from build123d import *

# Parameters (mm, degrees)
BOSS_EXTRUDE1_DEPTH = 4
SKETCH6_R           = 1.45
CUT_EXTRUDE1_DEPTH  = 63.610622102
SKETCH7_R           = 1.4
CUT_EXTRUDE2_DEPTH  = 64.549114864
FILLET1_R           = 1
FILLET2_R           = 0.5


with BuildPart() as part:
    # Sketch4 → Revolve1 (revolve)
    with BuildSketch(Plane(origin=(0, 0, 0), x_dir=(1, 0, 0), z_dir=(0, 1, 0)), mode=Mode.PRIVATE) as revolve1_sk:
        Polygon((9.95, -8.8), (0, -8.8), (0, 0), (12.5, 0), (12.5, -0.8), (11.5, -1.8), (9.95, -1.8), align=None)
    revolve1 = revolve(revolve1_sk.sketch.rotate(Axis((0, 0, 0), (0, 0, 1)), 180), axis=Axis((0, 0, 0), (0, 0, 1)))

    # Sketch5 → Boss-Extrude1 (add)
    with BuildSketch(Plane.XY):
        with BuildLine():
            Line((0, 12.5), (-60, 12.5))
            Line((-60, 12.5), (-60, -12.5))
            Line((-60, -12.5), (0, -12.5))
            ThreePointArc((0, -12.5), (12.5, 0), (0, 12.5))
        make_face()
    boss_extrude1 = extrude(amount=-BOSS_EXTRUDE1_DEPTH)

    # Sketch6 → Cut-Extrude1 (cut, through all)
    with BuildSketch(Plane.XY.offset(8.8)):
        with Locations((0, 6.5)):
            Circle(SKETCH6_R)
        with Locations((6.5, 0)):
            Circle(SKETCH6_R)
        with Locations((0, -6.5)):
            Circle(SKETCH6_R)
        with Locations((-6.5, 0)):
            Circle(SKETCH6_R)
    cut_extrude1 = extrude(amount=-CUT_EXTRUDE1_DEPTH, mode=Mode.SUBTRACT)

    # Mirror1: Revolve1, Boss-Extrude1, Cut-Extrude1 across plane
    add(revolve1.mirror(Plane.XY.offset(-4)))
    add(boss_extrude1.mirror(Plane.XY.offset(-4)))
    add(cut_extrude1.mirror(Plane.XY.offset(-4)), mode=Mode.SUBTRACT)

    # Sketch7 → Cut-Extrude2 (cut, through all)
    with BuildSketch(Plane.XY):
        with Locations((-55, 7.5)):
            Circle(SKETCH7_R)
        with Locations((-55, -7.5)):
            Circle(SKETCH7_R)
        with Locations((-40, 7.5)):
            Circle(SKETCH7_R)
        with Locations((-40, -7.5)):
            Circle(SKETCH7_R)
        with Locations((-25, 7.5)):
            Circle(SKETCH7_R)
        with Locations((-25, -7.5)):
            Circle(SKETCH7_R)
    extrude(amount=-CUT_EXTRUDE2_DEPTH, mode=Mode.SUBTRACT)

    # Fillet1
    fillet1_edges = [part.edges().sort_by_distance(p)[0] for p in [
        (-60, -12.5, -2),
        (-60, 12.5, -2),
    ]]
    fillet(fillet1_edges, radius=FILLET1_R)

    # Fillet2
    fillet2_edges = [part.edges().sort_by_distance(p)[0] for p in [
        (9.95, 0, -16.8),
        (9.95, 0, 8.8),
    ]]
    fillet(fillet2_edges, radius=FILLET2_R)


solid = part.part
Work out the finished part from the listing and answer in its coordinate system (mm). A direction names the side the tool comes from. Round coordinates to 2 decimals unless told otherwise and drop trailing zeros. Order: outer loops, then holes, each group sorted by start corner. A loop starts at its lowest first (then second) coordinate and runs counter-clockwise, first axis right, second up. Notation, with made-up numbers: M 58.25,-13 L 77.25,-13 A18 ccw 77.25,6 Z; hole C -28,-31 d5. An arc over 180 degrees is marked long. Put each result on its own line as item: value. Start each with the question number.
Q1. Flat-ended cylindrical pins translate along their axes: pin 1 (3.5 mm diameter, centred on x = -25, y = 7.5, fed in from +Z); pin 2 (1.5 mm diameter, centred on x = -20.5, y = -1.5, fed in from -Z); pin 3 (4 mm diameter, centred on y = 9.5, z = -13, fed in from +X). Find the tip coordinate at first contact, or state that the pin passes through.
Q2. A tool of negligible diameter and unlimited length cuts with its end or side. For faces 5 (the flat face through (5, -9, 1.8)), 6 (the cylindrical face through (-38.71, -8.04, -3.94)), from which of +Z, -Z, +X, -X, +Y, -Y can it reach the whole face along a straight path? Write none if from no direction.
Q3. Section A-A, the plane x = -40 is taken. Write down the section's boundary in (y, z), and give its area (3 significant figures).
Q4. Straight lines are drawn through the part: L1, parallel to Y at x = -55, z = -3.5; L2, parallel to Z at x = -50, y = -6; L3, parallel to X at y = 5.75, z = -10.75. For each, find the intervals that lie inside material, in ascending order. Write a range as [from, to].
Q5. Section B-B, the plane y = 0 is taken. Give the number of separate pieces and of enclosed holes in the cut face, and give its area (3 significant figures).
Q6. Section D-D, the plane z = -10.75 is taken. Write down the section's boundary in (x, y), and give its area (3 significant figures).
Q7. For a pull along Y with two mould halves and no side action, classify faces 1 (the cylindrical face through (7.9, 6.05, -13.1)), 2 (the cylindrical face through (-53.665, 7.921, -3.944)), 3 (the cylindrical face through (-23.71, 6.96, -3.94)), 4 (the flat face through (5, -9, -9.8)) as pulls with the +Y half, pulls with the -Y half, needs draft (parallel to the pull), parting line crosses it, or undercut.
Findings below:
1. pin 1: stops at z = 0
1. pin 2: stops at z = -8
1. pin 3: stops at x = 6.54
2. face 5: +Z
2. face 6: +Z, -Z
3. outline: M -12.5,-8 L -8.9,-8 L -8.9,0 L -12.5,0 Z; M -6.1,-8 L 6.1,-8 L 6.1,0 L -6.1,0 Z; M 8.9,-8 L 12.5,-8 L 12.5,0 L 8.9,0 Z
3. area: 155 mm^2
4. L1: y = [-12.5, -8.9], [-6.1, 6.1], [8.9, 12.5]
4. L2: z = [-8, 0]
4. L3: x = [-8.12, -1.24], [1.24, 8.12]
5. separate pieces: 3
5. enclosed holes: 0
5. area: 798 mm^2
6. outline: C 0,0 d19.9; hole C -6.5,0 d2.9; hole C 0,-6.5 d2.9; hole C 0,6.5 d2.9; hole C 6.5,0 d2.9
6. area: 285 mm^2
7. face 1: parting line crosses it
7. face 2: undercut
7. face 3: undercut
7. face 4: needs draft
